Input: part model. Units: mm. Frame: model coordinates. A direction names the side the tool comes from. Coordinates: 2 decimals unless noted, no trailing zeros. Order: outer loops, then holes, each group sorted by start corner. A loop starts at its lowest first (then second) coordinate and runs counter-clockwise, first axis right, second up. Notation, with made-up numbers: (-8.75, -31) -> (18.25, -31) arc R25 ccw to (18.25, -3) -> close; hole circle Ø10 at (45.5, 69). An arc over 180 degrees is marked (long way). Use one line per item in the form item = value. Start each with the question number.
1) Access query for faces 5 (the flat face through (-9.18, 1.52, -9.34)), 6 (the cylindrical face through (8.99, 1.52, 5.23)), 7 (the cylindrical face through (-3, 9, 0)), 8 (the flat face through (-3.5, 2, 13)), 9 (the flat face through (0, 0, 3)). Directions: +Z, -Z, +X, -X, +Y, -Y. A direction counts if a zero-diameter tool reaches every point of the face in a straight line with its end or side. Return the directions, or none.
2) Draft query along Z for faces 1 (the flat face through (12.68, 1.52, -3.28)), 2 (the cylindrical face through (12.04, 1.52, 1.57)), 3 (the cylindrical face through (-4.66, 1.52, -11.21)), 4 (the cylindrical face through (0.1, 1.5, 8.5)). Return one class per face: pulls with the +Z half, pulls with the -Z half, needs draft (parallel to the pull), parting line crosses it, or undercut.
3) Section query D-D on y = 13.75. Output: boundary loops of the cut face in (x, z), then the cut area to 3 significant figures.
4) Section query A-A on z = 0. Output: boundary loops of the cut face in (x, y).
5) Pin query (flat end, axial travel): pin 1 (2 mm diameter, centred on x = 7, z = -2.5, fed in from +Y); pin 2 (0.6 mm diameter, centred on y = 1, z = 12.5, fed in from +X); pin 3 (4 mm diameter, centred on x = -0.5, y = 13.5, fed in from +Z). Return the tip coordinate at first contact, or that it passes through.
6) Section query C-C on y = 2.25. Count the separate pieces of the cut face and the enclosed holes in it, then the cut area to 3 significant figures.
7) Ray query, line 1 along Z through (x, y) = (0, 5); line 2 along Z through (x, y) = (7.75, 2.25). Return the intervals inside material, ascending.
8) Section query B-B on x = 0. Output: boundary loops of the cut face in (y, z).
Autodesk Inventor part; units mm, degrees
ref_plane "YZ Plane" through (0, 0, 0) normal (1, 0, 0) x (0, 1, 0)
ref_plane "XZ Plane" through (0, 0, 0) normal (0, 1, 0) x (-1, 0, 0)
ref_plane "XY Plane" through (0, 0, 0) normal (0, 0, 1) x (1, 0, 0)
sketch "Sketch1" plane through (0, 0, 0) normal (0, 1, 0) x (-1, 0, 0)
  circle A0 centre (0, 0) radius 15
  dimension "d0" = 30
extrude "Extrusion1" add sketch "Sketch1" along normal blind 3
sketch "Sketch6" plane through (0, 3, 0) normal (0, 1, 0) x (1, 0, 0)
  circle A0 centre (0, 0) radius 3
  dimension "d24" = 6
extrude "Extrusion4" add sketch "Sketch6" along normal blind 12
sketch "Sketch8" plane through (0, 15, 0) normal (0, 1, 0) x (1, 0, 0)
  point P0 (0, 0)
  point P1 (0, 0)
hole "Hole2" at (0, 15, 0) direction (0, -1, 0) diameter 3.242 end through all
sketch "Sketch9" plane through (0, 3, 0) normal (0, 1, 0) x (1, 0, 0)
  arc A0 (3.1058, 11.5911) -> (-3.1058, 11.5911) centre (0, 0) ccw construction
  arc A1 (3.5199, 13.1366) -> (-3.5199, 13.1366) centre (0, 0) ccw
  arc A2 (2.6917, 10.0456) -> (-2.6917, 10.0456) centre (0, 0) ccw
  arc A3 (2.6917, 10.0456) -> (3.5199, 13.1366) centre (3.1058, 11.5911) ccw
  arc A4 (-3.5199, 13.1366) -> (-2.6917, 10.0456) centre (-3.1058, 11.5911) ccw
  circle A5 centre (0, 0) radius 15
  point P0 (0, 15)
  dimension "d37" = 3.2
  dimension "d38" = 30
  dimension "d39" = 15
  dimension "d45" = 12
extrude "Extrusion6" cut sketch "Sketch9" against normal through all contours A3 A2 A4 A1
pattern_circular "Circular Pattern2" count 3 over 360 about axis through (0, 3, 0) along (0, 1, 0) of "Extrusion6"
sketch "Sketch11" plane through (0, 3, 0) normal (0, 1, 0) x (1, 0, 0)
  circle A0 centre (0, -12) radius 3.5
  line L0 (3.5, -12) -> (3.5, -14.586)
  line L1 (-3.5, -12) -> (-3.5, -14.586)
  arc A1 (-3.5, -14.586) -> (3.5, -14.586) centre (0, 0) ccw
  circle A2 centre (0, 0) radius 15
  point P0 (-2.011, -14.8646)
  point P1 (2.011, -14.8646)
  dimension "d48" = 7
  dimension "d49" = 12
extrude "Extrusion7" cut sketch "Sketch11" against normal through all contours A0 A1 | L0 A1 A0 | A0 A1 L1 | A0 A1
fillet "Fillet1" radius 1 2 edges at (-3.5, 1.5, 14.586) (3.5, 1.5, 14.586)
pattern_circular "Circular Pattern3" count 3 over 360 about axis through (0, 0, 0) along (0, 1, 0) of "Extrusion7", "Fillet1"
properties part number "FrameSupport-Flange" material "Copper"
Answers below:
q1.face_5 = -X, +Y, -Y
q1.face_6 = +Y, -Y
q1.face_7 = +Y
q1.face_8 = +Z, +Y, -Y
q1.face_9 = +Z, -Z, +X, -X, -Y
q2.face_1 = pulls with the -Z half
q2.face_2 = undercut
q2.face_3 = undercut
q2.face_4 = pulls with the +Z half
q3.outline = circle Ø6 at (0, 0); hole circle Ø3.24 at (0, 0)
q3.area = 20.0 mm^2
q4.outline = (-15, 0) -> (-1.62, 0) -> (-1.62, 15) -> (-3, 15) -> (-3, 3) -> (-15, 3) -> close; (1.62, 0) -> (15, 0) -> (15, 3) -> (3, 3) -> (3, 15) -> (1.62, 15) -> close
q5.pin_1 = 3
q5.pin_2 = 8.73
q5.pin_3 = 3
q6.separate_pieces = 1
q6.enclosed_holes = 4
q6.area = 494 mm^2
q7.line_1 = -3 to -1.62, 1.62 to 3
q7.line_2 = -12.84 to -8.3, -3.7 to 6.94, 9.91 to 12.84
q8.outline = (0, -15) -> (3, -15) -> (3, -13.6) -> (0, -13.6) -> close; (0, -10.4) -> (3, -10.4) -> (3, -3) -> (15, -3) -> (15, -1.62) -> (0, -1.62) -> close; (0, 1.62) -> (15, 1.62) -> (15, 3) -> (3, 3) -> (3, 8.5) -> (0, 8.5) -> close
